from build123d import *

# Parameters (mm, degrees)
SKETCH_1_R      = 1.3
EXTRUDE_1_DEPTH = 6
SKETCH_2_W      = 3.381536624
SKETCH_2_H      = 1
EXTRUDE_2_DEPTH = 18
FILLET_1_R      = 2


with BuildPart() as part:
    # Эскиз1 → Бобышка-Вытянуть1 (new body)
    with BuildSketch(Plane(origin=(0, 0, 0), x_dir=(1, 0, 0), z_dir=(0, 1, 0))):
        with BuildLine():
            Line((-1.690768312, 1.975171515), (1.690768312, 1.975171515))
            ThreePointArc((1.690768312, 1.975171515), (0, -2.6), (-1.690768312, 1.975171515))
        make_face()
        with Locations(Location((0, 0, 0), (0, 0, 270))):
            Circle(SKETCH_1_R, mode=Mode.SUBTRACT)
    extrude(amount=EXTRUDE_1_DEPTH)

    # Эскиз2 → Бобышка-Вытянуть2 (add)
    with BuildSketch(Plane.XZ):
        with Locations((0, -2.475171515)):
            Rectangle(SKETCH_2_W, SKETCH_2_H)
    extrude(amount=-EXTRUDE_2_DEPTH)

    # Скругление1
    fillet_1_edges = [part.edges().sort_by_distance(p)[0] for p in [
        (-1.690768312, 3, -1.975171515),
        (1.690768312, 3, -1.975171515),
    ]]
    fillet(fillet_1_edges, radius=FILLET_1_R)


solid = part.part
Check sheet for the modelled part. Datum: model origin and axes. Units: mm. A direction names the side the tool comes from. Coordinates: 2 decimals unless noted, no trailing zeros. Write each loop counter-clockwise with the first axis right and the second up, starting at its lowest first coordinate (ties: lowest second). Pieces come first, ordered by that corner, then holes. Notation, with made-up numbers: M 78,-29 L 111,-29 A35 ccw 111,9 Z; hole C 69,-34 d5. An arc over 180 degrees is marked long. Answer as CSV lines item,"result".
Q1. Cross-section at D-D (x = 1.1). Record the boundary of the cut face in (y, z), then the cut area to 3 significant figures.
Check result:
outline,"M 0,-2.98 L 18,-2.98 L 18,-1.98 L 6,-1.98 L 6,-0.69 L 0,-0.69 Z; M 0,0.69 L 6,0.69 L 6,2.36 L 0,2.36 Z"
area,"35.7 mm^2"
Q2. Cross-section at A-A (x = 0). Record the boundary of the cut face in (y, z), then the cut area to 3 significant figures.
Check result:
outline,"M 0,-2.98 L 18,-2.98 L 18,-1.98 L 6,-1.98 L 6,-1.3 L 0,-1.3 Z; M 0,1.3 L 6,1.3 L 6,2.6 L 0,2.6 Z"
area,"29.9 mm^2"
Q3. Go/stop test with flat-tipped pins: pin 1 (3 mm diameter, centred on x = 1.5, y = 10.5, fed in from +Z); pin 2 (0.5 mm diameter, centred on y = 10, z = -2.5, fed in from -X); pin 3 (0.5 mm diameter, centred on y = 7, z = -2.5, fed in from +X). Record where each tip stops, or that it passes through.
Check result:
pin 1,"z = -1.98"
pin 2,"x = -1.69"
pin 3,"x = 1.69"
Q4. Cross-section at C-C (y = 1.25). Record the boundary of the cut face in (x, z).
Check result:
outline,"M -2.09,-1.55 A2 cw -1.69,-2.75 L -1.69,-2.98 L 1.69,-2.98 L 1.69,-2.75 A2 cw 2.09,-1.55 A2.6 ccw long Z; hole C 0,0 d2.6"
Q5. Set-up check for faces 1 (the face through (-1.789, 3.042, -2.125)), 2 (the face through (0, 12, -1.975)): record each of +Z, -Z, +X, -X, +Y, -Y from which the full face is reachable in a straight line by a thin tool's end or side.
Check result:
face 1,"-Z, -X, +Y, -Y"
face 2,"+Z, +X, -X, +Y"
Q6. Material ranges on probe 1 along X at (y, z) = (2.85, 0); probe 2 along Z at (x, y) = (-1.1, 13.25); probe 3 along Z at (x, y) = (0.8, 4), recorded low to high. Write a range as from..to.
Check result:
probe 1,"-2.6..-1.3, 1.3..2.6"
probe 2,"-2.98..-1.98"
probe 3,"-2.98..-1.02, 1.02..2.47"
Q7. Cross-section at B-B (z = 0.95). Record the boundary of the cut face in (x, y).
Check result:
outline,"M -2.42,0 L -0.89,0 L -0.89,6 L -2.42,6 Z; M 0.89,0 L 2.42,0 L 2.42,6 L 0.89,6 Z"
Q8. Mould release check, pull along Z, two halves, no side actions. Record for faces 3 (the face through (-1.691, 10.9, -2.5)), 4 (the face through (0, 9, -2.975)), 5 (the face through (0.39, 2.96, 1.24)): released by +Z, released by -Z, zero draft, split by the parting line, or undercut.
Check result:
face 3,"zero draft"
face 4,"released by -Z"
face 5,"undercut"
